Drawing for the job (mm, zero at the part's lowest x, y, z). A direction names the side the tool comes from. Give positions to 0.01 mm unless a question says otherwise; leave off trailing zeros. Loops run counter-clockwise (first coordinate to the right, second up) from the corner with the lowest first, then second, coordinate; pieces in that order, holes last. Notation, with made-up numbers: (57.25, -9) - (81.25, -9) arc R23 cw to (81.25, 28) - close; hole circle Ø11 at (17, 35). An arc over 180 degrees is marked (long way). Return JSON: item names as keys, results as strings. Group by question number.
1) Slice it at A-A (z = 3.5). List the corners of the cut face in (x, y).
2) Drop flat-ended pins along their axis: pin 1 (3.5 mm diameter, centred on y = 3.5, z = 4.5, fed in from -X); pin 2 (1.8 mm diameter, centred on x = 56.5, z = 18.5, fed in from -Y); pin 3 (1.2 mm diameter, centred on x = 54, z = 3, fed in from +Y); pin 4 (10 mm diameter, centred on x = 50.5, z = 16.5, fed in from -Y). Give the stop position or say it passes through.
3) Slice it at C-C (x = 7). List the corners of the cut face in (y, z), and give its area (3 significant figures).
4) Slice it at D-D (y = 3). List the corners of the cut face in (x, z), and give its area (3 significant figures).
5) Slice it at B-B (y = 11). List the corners of the cut face in (x, z).
6) Drill centre lines: probe 1 along X at (y, z) = (9.9, 3.5); probe 2 along X at (y, z) = (1.15, 18.5); probe 3 along Y at (x, z) = (42, 14). Where is each one in solid material? Low to high. Write a range as from..to.
7) 3-axis set-ups, long thin cutter, end or side, ignore diameter. For the marked faces 1, 2, 3, 4 and 5: which of +Z, -Z, +X, -X, +Y, -Y reach the whole face in a straight line?
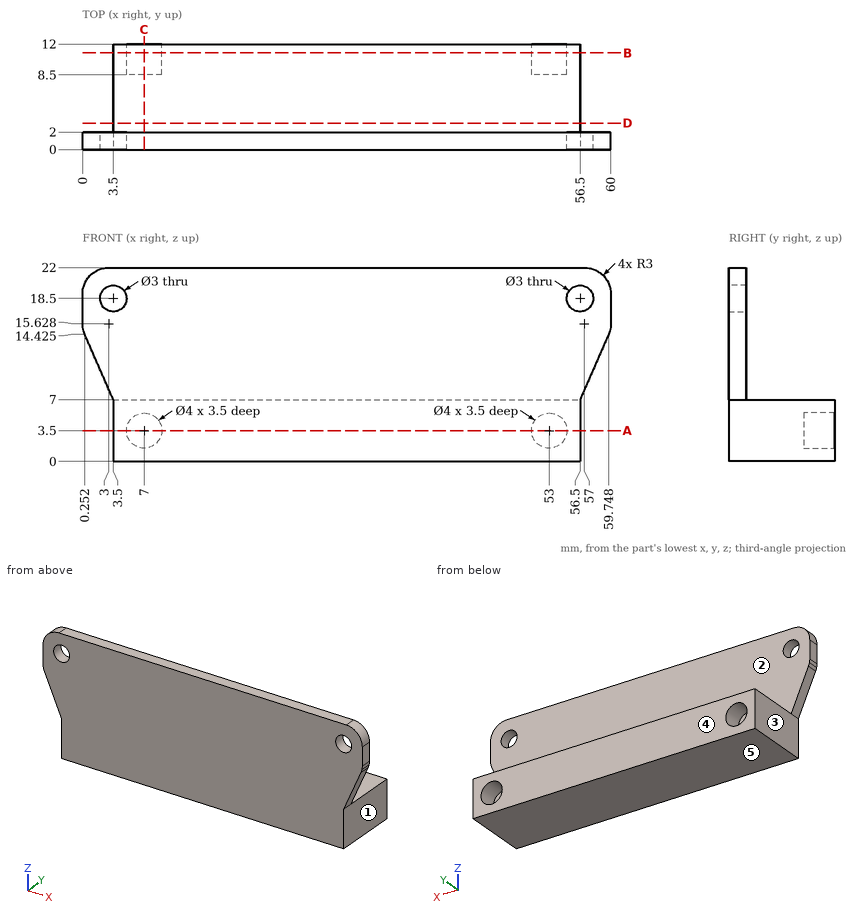
Results:
{
 "1": {"outline": "(3.5, 0) - (56.5, 0) - (56.5, 12) - (55, 12) - (55, 8.5) - (51, 8.5) - (51, 12) - (9, 12) - (9, 8.5) - (5, 8.5) - (5, 12) - (3.5, 12) - close"},
 "2": {"pin 1": "x = 3.5", "pin 2": "through", "pin 3": "y = 8.5", "pin 4": "y = 0"},
 "3": {"outline": "(0, 0) - (12, 0) - (12, 1.5) - (8.5, 1.5) - (8.5, 5.5) - (12, 5.5) - (12, 7) - (2, 7) - (2, 22) - (0, 22) - close", "area": "100 mm2"},
 "4": {"outline": "(3.5, 0) - (56.5, 0) - (56.5, 7) - (3.5, 7) - close", "area": "371 mm2"},
 "5": {"outline": "(3.5, 0) - (56.5, 0) - (56.5, 7) - (3.5, 7) - close; hole circle Ø4 at (7, 3.5); hole circle Ø4 at (53, 3.5)"},
 "6": {"probe 1": "3.5..5, 9..51, 55..56.5", "probe 2": "0..2, 5..55, 58..60", "probe 3": "0..2"},
 "7": {"face 1": "-Z, +X, +Y, -Y", "face 2": "+Z, +X, -X, +Y", "face 3": "-Z, -X, +Y, -Y", "face 4": "+Z, -Z, +X, -X, +Y", "face 5": "-Z, +X, -X, +Y, -Y"}
}
